Could you check a few things on this model? Use its own coordinates, in mm. Give positions to 0.01 mm unless a question says otherwise; leave off trailing zeros. Write each loop counter-clockwise with the first axis right and the second up, starting at its lowest first coordinate (ties: lowest second). Pieces come first, ordered by that corner, then holes. Notation, with made-up numbers: (88.5, 81) -> (141.5, 81) arc R24 cw to (141.5, 107) -> close; hole circle Ø3 at (84, -16.5). An arc over 180 degrees is marked (long way). Write item = value, one per line. Start each with the question number.
```python
from build123d import *

# Parameters (mm, degrees)
SKETCH3_W           = 92
SKETCH3_H           = 31
BOSS_EXTRUDE2_DEPTH = 5
SKETCH4_R           = 103
SKETCH4_R_2         = 73
CUT_EXTRUDE1_DEPTH  = 49.79805324
SKETCH5_R           = 2.15
CUT_EXTRUDE2_DEPTH  = 49.79805324
CUT_EXTRUDE4_DEPTH  = 56.695601263
SKETCH8_R           = 1.2
CUT_EXTRUDE5_DEPTH  = 49.79805324
SKETCH9_R           = 2.1
CUT_EXTRUDE6_DEPTH  = 3.4
SKETCH10_W          = 20
SKETCH10_H          = 6
CUT_EXTRUDE7_DEPTH  = 49.79805324
FILLET1_R           = 2


with BuildPart() as part:
    # Sketch3 → Boss-Extrude2 (new body)
    with BuildSketch(Plane.XY):
        Rectangle(SKETCH3_W, SKETCH3_H)
    extrude(amount=BOSS_EXTRUDE2_DEPTH)

    # Sketch4 → Cut-Extrude1 (cut, through all)
    with BuildSketch(Plane.XY.offset(5)):
        with Locations((0, -53.5)):
            Circle(SKETCH4_R)
        with Locations((0, -53.5)):
            Circle(SKETCH4_R_2, mode=Mode.SUBTRACT)
    extrude(amount=-CUT_EXTRUDE1_DEPTH, mode=Mode.SUBTRACT)

    # Sketch5 → Cut-Extrude2 (cut, through all)
    with BuildSketch(Plane.XY.offset(5)):
        with Locations((38, -7.5)):
            Circle(SKETCH5_R)
        with Locations(Location((-38, -7.5, 0), (0, 0, 180))):
            Circle(SKETCH5_R)
    extrude(amount=-CUT_EXTRUDE2_DEPTH, mode=Mode.SUBTRACT)

    # Sketch7 → Cut-Extrude4 (cut, through all)
    with BuildSketch(Plane.XZ.offset(15.5)):
        Polygon((-1, 0), (0, 1.6), (1, 0), align=None)
    extrude(amount=-CUT_EXTRUDE4_DEPTH, mode=Mode.SUBTRACT)

    # Sketch8 → Cut-Extrude5 (cut, through all)
    with BuildSketch(Plane.XY.offset(5)):
        with Locations((-32, 7.5)):
            Circle(SKETCH8_R)
        with Locations((32, 7.5)):
            Circle(SKETCH8_R)
    extrude(amount=-CUT_EXTRUDE5_DEPTH, mode=Mode.SUBTRACT)

    # Sketch9 → Cut-Extrude6 (cut)
    with BuildSketch(Plane(origin=(0, 0, 0), x_dir=(-1, 0, 0), z_dir=(0, 0, -1))):
        with Locations((32, 7.5)):
            Circle(SKETCH9_R)
        with Locations((-32, 7.5)):
            Circle(SKETCH9_R)
    extrude(amount=-CUT_EXTRUDE6_DEPTH, mode=Mode.SUBTRACT)

    # Sketch10 → Cut-Extrude7 (cut, through all)
    with BuildSketch(Plane(origin=(0, 0, 0), x_dir=(-1, 0, 0), z_dir=(0, 0, -1))):
        with Locations((10.5, -4.5)):
            Rectangle(SKETCH10_W, SKETCH10_H)
    extrude(amount=-CUT_EXTRUDE7_DEPTH, mode=Mode.SUBTRACT)

    # Fillet1
    # the kernel refuses this fillet: 2 mm, written as the material it takes off along each edge
    with BuildSketch(Plane(origin=(-20.5, -7.5, 0), x_dir=(0, -1, 0), z_dir=(1, 0, 0))) as fillet1_piece_1_section:
        with BuildLine():
            CenterArc((FILLET1_R, -FILLET1_R), FILLET1_R, 90, 90)
            Line((0, -FILLET1_R), (0, 0))
            Line((0, 0), (FILLET1_R, 0))
        make_face()
    fillet1_piece_1 = extrude(amount=24.5, mode=Mode.PRIVATE)
    fillet1_piece_1 = split(fillet1_piece_1, bisect_by=Plane(origin=(-0.5, -7.952790229, 0.452790229), z_dir=(-1, 0, 0)), keep=Keep.TOP, mode=Mode.PRIVATE)
    add(fillet1_piece_1, mode=Mode.SUBTRACT)
    with BuildSketch(Plane(origin=(-20.5, -1.5, 0), x_dir=(-1, 0, 0), z_dir=(0, -1, 0))) as fillet1_piece_2:
        with BuildLine():
            CenterArc((FILLET1_R, -FILLET1_R), FILLET1_R, 90, 90)
            Line((0, -FILLET1_R), (0, 0))
            Line((0, 0), (FILLET1_R, 0))
        make_face()
    extrude(amount=6, mode=Mode.SUBTRACT)
    with BuildSketch(Plane(origin=(4, -1.5, 0), x_dir=(0, 1, 0), z_dir=(-1, 0, 0))) as fillet1_piece_3_section:
        with BuildLine():
            CenterArc((FILLET1_R, -FILLET1_R), FILLET1_R, 90, 90)
            Line((0, -FILLET1_R), (0, 0))
            Line((0, 0), (FILLET1_R, 0))
        make_face()
    fillet1_piece_3 = extrude(amount=24.5, mode=Mode.PRIVATE)
    fillet1_piece_3 = split(fillet1_piece_3, bisect_by=Plane(origin=(-0.5, -1.047209771, 0.452790229), z_dir=(-1, 0, 0)), keep=Keep.TOP, mode=Mode.PRIVATE)
    add(fillet1_piece_3, mode=Mode.SUBTRACT)
    with BuildSketch(Plane(origin=(-25.5, -7.5, 0), x_dir=(0, -1, 0), z_dir=(1, 0, 0))) as fillet1_piece_4a_section:
        with BuildLine():
            CenterArc((FILLET1_R, -FILLET1_R), FILLET1_R, 90, 90)
            Line((0, -FILLET1_R), (0, 0))
            Line((0, 0), (FILLET1_R, 0))
        make_face()
    fillet1_piece_4a = extrude(amount=29.5, mode=Mode.PRIVATE)
    fillet1_piece_4a = split(fillet1_piece_4a, bisect_by=Plane(origin=(-20.5, -7.952790229, 0.452790229), z_dir=(-1, 0, 0)), keep=Keep.TOP, mode=Mode.PRIVATE)
    with BuildSketch(Plane(origin=(-20.5, -1.5, 0), x_dir=(-1, 0, 0), z_dir=(0, -1, 0))) as fillet1_piece_4b_section:
        with BuildLine():
            CenterArc((FILLET1_R, -FILLET1_R), FILLET1_R, 90, 90)
            Line((0, -FILLET1_R), (0, 0))
            Line((0, 0), (FILLET1_R, 0))
        make_face()
    fillet1_piece_4b = extrude(amount=11, mode=Mode.PRIVATE)
    fillet1_piece_4b = split(fillet1_piece_4b, bisect_by=Plane(origin=(-20.952790229, -7.5, 0.452790229), z_dir=(0, -1, 0)), keep=Keep.TOP, mode=Mode.PRIVATE)
    fillet1_piece_4 = fillet1_piece_4a & fillet1_piece_4b
    add(fillet1_piece_4, mode=Mode.SUBTRACT)
    with BuildSketch(Plane(origin=(-20.5, 3.5, 0), x_dir=(-1, 0, 0), z_dir=(0, -1, 0))) as fillet1_piece_5a_section:
        with BuildLine():
            CenterArc((FILLET1_R, -FILLET1_R), FILLET1_R, 90, 90)
            Line((0, -FILLET1_R), (0, 0))
            Line((0, 0), (FILLET1_R, 0))
        make_face()
    fillet1_piece_5a = extrude(amount=11, mode=Mode.PRIVATE)
    fillet1_piece_5a = split(fillet1_piece_5a, bisect_by=Plane(origin=(-20.952790229, -1.5, 0.452790229), z_dir=(0, 1, 0)), keep=Keep.TOP, mode=Mode.PRIVATE)
    with BuildSketch(Plane(origin=(4, -1.5, 0), x_dir=(0, 1, 0), z_dir=(-1, 0, 0))) as fillet1_piece_5b_section:
        with BuildLine():
            CenterArc((FILLET1_R, -FILLET1_R), FILLET1_R, 90, 90)
            Line((0, -FILLET1_R), (0, 0))
            Line((0, 0), (FILLET1_R, 0))
        make_face()
    fillet1_piece_5b = extrude(amount=29.5, mode=Mode.PRIVATE)
    fillet1_piece_5b = split(fillet1_piece_5b, bisect_by=Plane(origin=(-20.5, -1.047209771, 0.452790229), z_dir=(-1, 0, 0)), keep=Keep.TOP, mode=Mode.PRIVATE)
    fillet1_piece_5 = fillet1_piece_5a & fillet1_piece_5b
    add(fillet1_piece_5, mode=Mode.SUBTRACT)


solid = part.part
```
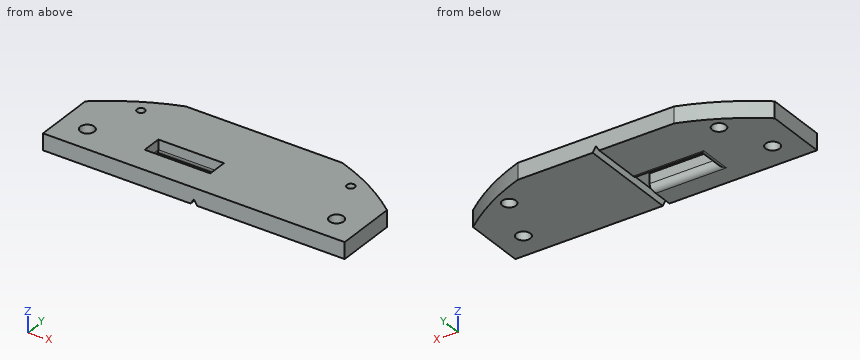
(1) Imagine slicing it at D-D (x = -27). Please give me the cut outline in (y, z), then the cut area to 3 significant figures.
(2) Imagine slicing it at C-C (x = -9.5). Please give me the cut outline in (y, z), then the cut area to 3 significant figures.
(3) If I drill on line 1 along X through (y, z) = (9, 3); line 2 along Y through (x, z) = (-3, 3.1); line 3 along X through (y, z) = (-6.5, 3.95), over which ranges is the centre line in solid material (lowest first)? Write a range as from..to.
(4) Imagine slicing it at A-A (x = 32). Please give me the cut outline in (y, z), then the cut area to 3 significant figures.
(5) I'm going to push flat-ended pins straight in: pin 1 (3 mm diameter, centred on x = 32, y = 7.5, fed in from -Z); pin 2 (3.5 mm diameter, centred on x = 32, y = 8.5, fed in from -Z); pin 3 (4 mm diameter, centred on x = 38, y = -7.5, fed in from -Z). Where does each tip first touch, or does it pass through?
(6) Imagine slicing it at B-B (y = 7.5). Please give me the cut outline in (x, z), then the cut area to 3 significant figures.
Answers below:
q1.outline = (-15.5, 0) -> (14.32, 0) -> (14.32, 5) -> (-15.5, 5) -> close
q1.area = 149 mm^2
q2.outline = (-15.5, 0) -> (-9.5, 0) arc R2 ccw to (-7.5, 2) -> (-7.5, 5) -> (-15.5, 5) -> close; (-1.5, 2) arc R2 ccw to (0.5, 0) -> (15.5, 0) -> (15.5, 5) -> (-1.5, 5) -> close
q2.area = 123 mm^2
q3.line_1 = -37.72..-33.47, -30.53..30.53, 33.47..37.72
q3.line_2 = -15.5..-7.5, -1.5..15.5
q3.line_3 = -46..-39.9, -36.1..-20.5, -0.5..36.1, 39.9..46
q4.outline = (-15.5, 0) -> (5.4, 0) -> (5.4, 3.4) -> (6.3, 3.4) -> (6.3, 5) -> (-15.5, 5) -> close; (8.7, 3.4) -> (9.6, 3.4) -> (9.6, 0) -> (12.11, 0) -> (12.11, 5) -> (8.7, 5) -> close
q4.area = 120 mm^2
q5.pin_1 = 3.4
q5.pin_2 = 0
q5.pin_3 = through
q6.outline = (-40.1, 0) -> (-34.1, 0) -> (-34.1, 3.4) -> (-33.2, 3.4) -> (-33.2, 5) -> (-40.1, 5) -> close; (-30.8, 3.4) -> (-29.9, 3.4) -> (-29.9, 0) -> (-1, 0) -> (0, 1.6) -> (1, 0) -> (29.9, 0) -> (29.9, 3.4) -> (30.8, 3.4) -> (30.8, 5) -> (-30.8, 5) -> close; (33.2, 3.4) -> (34.1, 3.4) -> (34.1, 0) -> (40.1, 0) -> (40.1, 5) -> (33.2, 5) -> close
q6.area = 363 mm^2
